Build history of the part. All positions in model axes, mm. Face numbers are marked on the shaded views. Give positions to 0.01 mm unless a question says otherwise; leave off trailing zeros. Order: outer loops, then holes, each group sorted by start corner. A loop starts at its lowest first (then second) coordinate and runs counter-clockwise, first axis right, second up. Notation, with made-up numbers: (22.25, -17) - (73.25, -17) arc R17 ccw to (73.25, -1) - close; hole circle Ø2 at (26.25, 2). An arc over 180 degrees is marked (long way). Write each question's results on one line, items separated by ' | '. Start each with the question number.
1) Cut at C-C on x = 47. List the corners of the cut face in (y, z) (3 decimals), plus the area to 3 significant figures.
2) Cut at A-A on y = 0. List the corners of the cut face in (x, z) (3 decimals), plus the area to 3 significant figures.
3) Drill centre lines: line 1 along Y through (x, z) = (78, 0) (3 decimals); line 2 along Y through (x, z) = (129.5, -13.5). Where is each one in solid material? Low to high. Write a range as from..to.
4) Drop flat-ended pins along their axis: pin 1 Ø2 at (x, y) = (82.5, 2) entering from +Z; pin 2 Ø1 at (x, z) = (182, -2) entering from +Y; pin 3 Ø6 at (x, y) = (183.5, -4.5) entering from -Z. Give the stop position or say it passes through.
5) Two-plate mould, pull along Y, no slides. Class the marked faces 1 and 2: +Y half, -Y half, draft (parallel to the pull), parting line (faces both ways), or undercut.
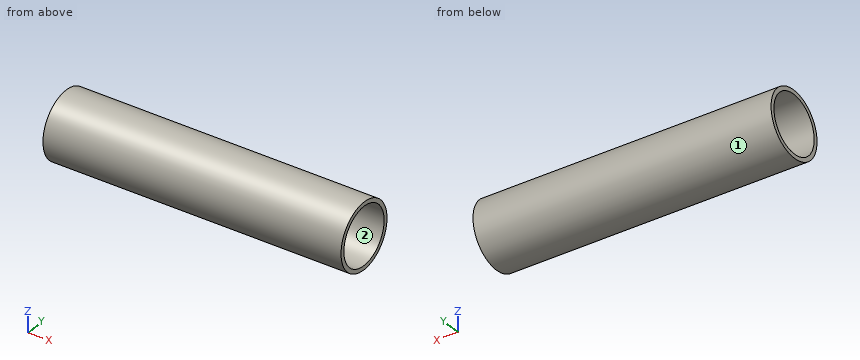
from build123d import *

# Parameters (mm, degrees)
F0_R      = 25.4
F1_DEPTH  = 254
F2_T      = -3.175
F1_FACE_R = 25.4
F3_DEPTH  = 25.4


with BuildPart() as f1:
    # F0 (on Right) → F1 (new body)
    with BuildSketch(Plane.YZ):
        Circle(F0_R)
    extrude(amount=F1_DEPTH)

    # F2
    f2_openings = [f1.faces().sort_by_distance(p)[0] for p in [
        (254, 0, 0),
    ]]
    offset(amount=F2_T, openings=f2_openings)

    # F1_face (on face) → F3 (cut)
    with BuildSketch(Plane(origin=(0, 0, 0), x_dir=(0, 1, 0), z_dir=(-1, 0, 0))):
        Circle(F1_FACE_R)
    extrude(amount=-F3_DEPTH, mode=Mode.SUBTRACT)


solid = f1.part
Results:
1) outline: circle Ø50.8 at (0, 0); hole circle Ø44.45 at (0, 0) | area: 475 mm^2
2) outline: (25.4, -25.4) - (254, -25.4) - (254, -22.225) - (25.4, -22.225) - close; (25.4, 22.225) - (254, 22.225) - (254, 25.4) - (25.4, 25.4) - close | area: 1,450 mm^2
3) line 1: -25.4..-22.225, 22.225..25.4 | line 2: -21.52..-17.66, 17.66..21.52
4) pin 1: z = 25.38 | pin 2: y = 25.36 | pin 3: z = -25.36
5) face 1: parting line | face 2: undercut
